Verification items for the finished model (mm, model axes). Coordinates: 2 decimals unless noted, no trailing zeros. Loops run counter-clockwise (first coordinate to the right, second up) from the corner with the lowest first, then second, coordinate; pieces in that order, holes last. Notation, with made-up numbers: (11.5, 27) -> (31.5, 27) arc R25 cw to (31.5, 54) -> close; hole circle Ø9 at (74, -32). An arc over 180 degrees is marked (long way). Use CSV: the item, a comma, the result in double quotes. Start each with the question number.
```python
from build123d import *
from build123d import SkipClean  # not in build123d's __all__

# Parameters (mm, degrees)
F0_R     = 35
F1_DEPTH = 50
F2_T     = -3
F6_DEPTH = 25
F7_R     = 5
F8_DEPTH = 25


# Not quite as in the source:
# - after a boolean that leaves OpenCascade's solid faulty, fix() repairs it


with BuildPart() as f1:
    # F0 (on Top) → F1 (new body)
    with BuildSketch(Plane.XY):
        Circle(F0_R)
    extrude(amount=F1_DEPTH)

    # F2
    f2_openings = [f1.faces().sort_by_distance(p)[0] for p in [
        (0, 0, 50),
    ]]
    offset(amount=F2_T, openings=f2_openings)

    # F3 (on Right) → F4 (revolve)
    with BuildSketch(Plane.YZ):
        Polygon((-27, 35), (-32, 35), (-32, 26.3397459622), align=None)
    revolve(axis=Axis((0, 0, 50.3253415227), (0, 0, 1)))

    # F5 (on face) → F6 (cut)
    with BuildSketch(Plane.XY.offset(35)):
        with BuildLine():
            ThreePointArc((-8.2822094433, 30.9096264413), (-25.3873068893, 19.4803657283), (-32, 0))
            Line((-32, 0), (0, 0))
            Line((0, 0), (-8.2822094433, 30.9096264413))
        make_face()
        with BuildLine():
            Line((0, 32), (0, 0))
            Line((0, 0), (30.9096264413, 8.2822094433))
            ThreePointArc((30.9096264413, 8.2822094433), (19.4803657283, 25.3873068893), (0, 32))
        make_face()
        with BuildLine():
            Line((32, 0), (0, 0))
            Line((0, 0), (8.2822094433, -30.9096264413))
            ThreePointArc((8.2822094433, -30.9096264413), (25.3873068893, -19.4803657283), (32, 0))
        make_face()
        with BuildLine():
            Line((0, -32), (0, 0))
            Line((0, 0), (-30.9096264413, -8.2822094433))
            ThreePointArc((-30.9096264413, -8.2822094433), (-19.4803657283, -25.3873068893), (0, -32))
        make_face()
    with SkipClean():  # cleaning this boolean's faces spoils the solid; the shape is the same uncleaned
        extrude(amount=-F6_DEPTH, mode=Mode.SUBTRACT)

    # F7 (on face) → F8 (cut)
    with BuildSketch(Plane.XY.offset(3)):
        Circle(F7_R)
    extrude(amount=-F8_DEPTH, mode=Mode.SUBTRACT)

    add(f1.part.fix(), mode=Mode.REPLACE)


solid = f1.part
```
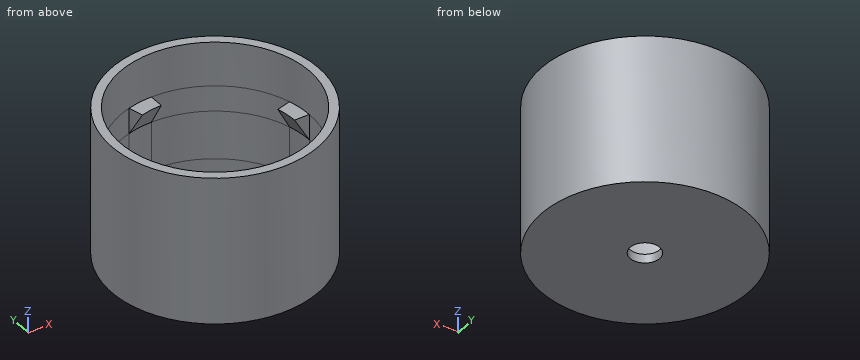
1. Depth check by flat-ended pin: pin 1 (3 mm diameter, centred on x = 7, z = 27, fed in from -Y); pin 2 (8 mm diameter, centred on x = 0, y = 0, fed in from +Z); pin 3 (1.5 mm diameter, centred on y = -28.5, z = 32.5, fed in from -X); pin 4 (2.5 mm diameter, centred on x = 30, z = 32, fed in from -Y). Enter the tip coordinate at first touch or a pass-through.
2. Cross-section at D-D, the plane z = 33. Record the boundary of the cut face in (x, y), plus the area to 3 significant figures.
3. Cross-section at C-C, the plane y = 16. Record the boundary of the cut face in (x, z), plus the area to 3 significant figures.
4. Cross-section at A-A, the plane z = 15. Record the boundary of the cut face in (x, y).
5. Cross-section at B-B, the plane x = 11. Record the boundary of the cut face in (y, z).
6. Scan lines: line 1 (Y direction, x = 0, z = 1.75); line 2 (Y direction, x = 0, z = 39.75); line 3 (Z direction, x = -23, y = -5.5). Record each from-to range of solid material in increasing order.
Solution:
1,pin 1,"stops at y = -34.57"
1,pin 2,"passes through"
1,pin 3,"stops at x = -21.33"
1,pin 4,"stops at y = -19.96"
2,outline,"circle Ø70 at (0, 0); hole (-32, 0) -> (-28.15, 0) arc R28.15 ccw to (-27.2, -7.29) -> (-30.91, -8.28) arc R32 ccw to (0, -32) -> (0, -28.15) arc R28.15 ccw to (7.29, -27.2) -> (8.28, -30.91) arc R32 ccw to (32, 0) -> (28.15, 0) arc R28.15 ccw to (27.2, 7.29) -> (30.91, 8.28) arc R32 ccw to (0, 32) -> (0, 28.15) arc R28.15 ccw to (-7.29, 27.2) -> (-8.28, 30.91) arc R32 ccw to start"
2,area,"753 mm2"
3,outline,"(-31.13, 0) -> (31.13, 0) -> (31.13, 50) -> (27.71, 50) -> (27.71, 3) -> (-27.71, 3) -> (-27.71, 50) -> (-31.13, 50) -> close"
3,area,"508 mm2"
4,outline,"circle Ø70 at (0, 0); hole circle Ø64 at (0, 0)"
5,outline,"(-33.23, 0) -> (33.23, 0) -> (33.23, 50) -> (30.05, 50) -> (30.05, 3) -> (-30.05, 3) -> (-30.05, 50) -> (-33.23, 50) -> close"
6,line 1,"y = -35 to -5, 5 to 35"
6,line 2,"y = -35 to -32, 32 to 35"
6,line 3,"z = 0 to 3"
